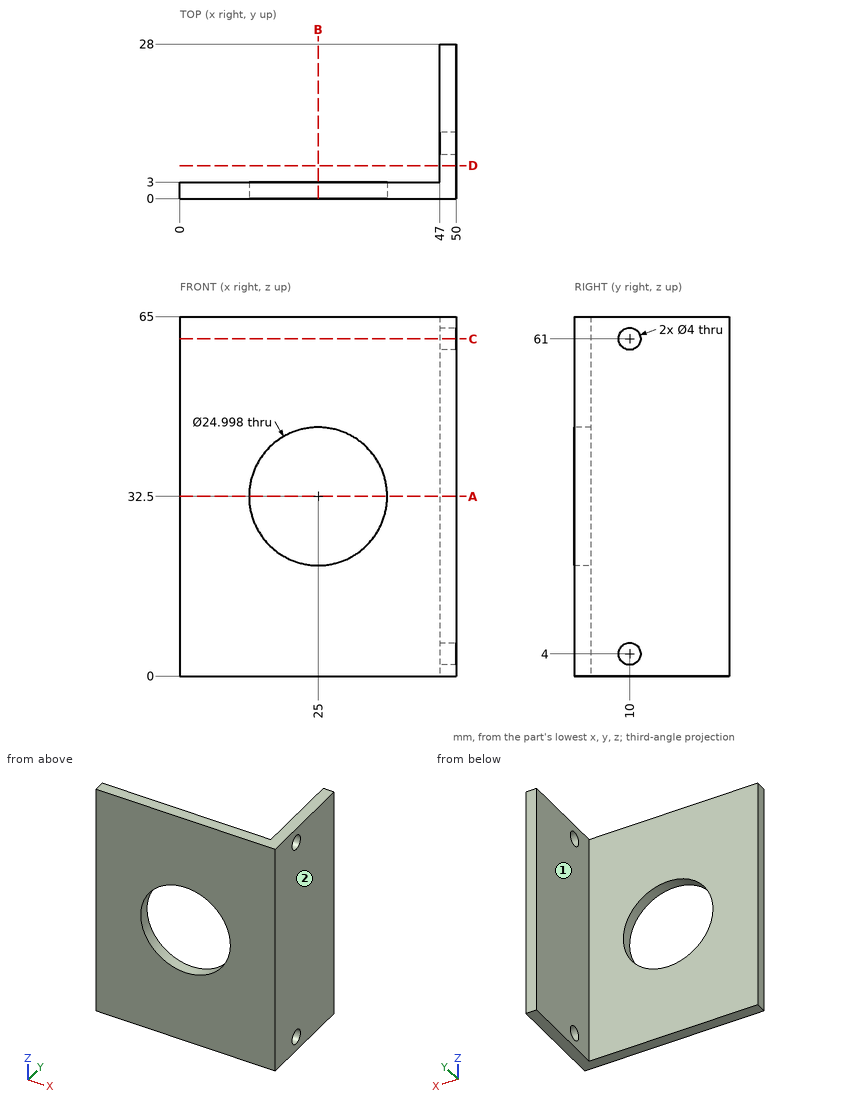
Drawing for the job (mm, zero at the part's lowest x, y, z). A direction names the side the tool comes from. Round coordinates to 2 decimals unless told otherwise and drop trailing zeros. Write each loop counter-clockwise with the first axis right and the second up, starting at its lowest first coordinate (ties: lowest second). Pieces come first, ordered by that corner, then holes. Notation, with made-up numbers: (28, 39.5) - (79, 39.5) arc R16 ccw to (79, 66.5) - close; hole circle Ø6 at (22.5, -11). An arc over 180 degrees is marked (long way). Write item = value, one per line. Start each with the question number.
Q1. Probe L1, parallel to Y at x = 48.7, z = 61; L2, parallel to X at y = 1.4, z = 32.5; L3, parallel to X at y = 12.5, z = 34. List the from-to ranges inside material, lowest first. Write a range as from..to.
Q2. Band-saw the part on A-A (z = 32.5). Give the cut face in (x, y).
Q3. Band-saw the part on C-C (z = 61). Give the cut face in (x, y).
Q4. Drop flat-ended pins along their axis: pin 1 (6 mm diameter, centred on y = 22, z = 25, fed in from -X); pin 2 (12 mm diameter, centred on x = 17.5, z = 50, fed in from +Y). Give the stop position or say it passes through.
Q5. Which spindle directions (+Z, -Z, +X, -X, +Y, -Y) get a long thin tool onto all of the face, cutting with end or side? Do the marked faces 1 and 2. Say none if no direction does.
Q6. Band-saw the part on B-B (x = 25). Give the cut face in (y, z), then the cut area to 3 significant figures.
Q7. Band-saw the part on D-D (y = 6). Give the cut face in (x, z).
Answers below:
q1.L1 = 0..8, 12..28
q1.L2 = 0..12.5, 37.5..50
q1.L3 = 47..50
q2.outline = (0, 0) - (12.5, 0) - (12.5, 3) - (0, 3) - close; (37.5, 0) - (50, 0) - (50, 28) - (47, 28) - (47, 3) - (37.5, 3) - close
q3.outline = (0, 0) - (50, 0) - (50, 8) - (47, 8) - (47, 3) - (0, 3) - close; (47, 12) - (50, 12) - (50, 28) - (47, 28) - close
q4.pin_1 = 47
q4.pin_2 = 3
q5.face_1 = +Z, -Z, -X, +Y
q5.face_2 = +Z, -Z, +X, +Y, -Y
q6.outline = (0, 0) - (3, 0) - (3, 20) - (0, 20) - close; (0, 45) - (3, 45) - (3, 65) - (0, 65) - close
q6.area = 120 mm2
q7.outline = (47, 0) - (50, 0) - (50, 65) - (47, 65) - close
